from build123d import *

# Parameters (mm, degrees)
CORTE_EXTRUS_O1_DEPTH      = 51.902259282
CORTE_EXTRUS_O1_DEPTH_BACK = 51.902259282
ESBO_O2_R                  = 4.25


with BuildPart() as part:
    # Esboço1 → Revolução1 (revolve)
    with BuildSketch(Plane(origin=(0, 0, 0), x_dir=(0, 0, -1), z_dir=(1, 0, 0))):
        Polygon((15.5, 35.2), (15.5, 0), (24.5, 0), (26, 1.5), (26, 22.5), (22.5, 22.5), (22.5, 35.2), align=None)
    revolve(axis=Axis((0, 0, 0), (0, 1, 0)))

    # Esboço2 → Corte-extrusão1 (cut, two sides: drawn at the far end of the back side and taken through both)
    with BuildSketch(Plane.XY.offset(-CORTE_EXTRUS_O1_DEPTH_BACK)):
        with Locations((0, 9.5)):
            Circle(ESBO_O2_R)
    extrude(amount=CORTE_EXTRUS_O1_DEPTH + CORTE_EXTRUS_O1_DEPTH_BACK, mode=Mode.SUBTRACT)


solid = part.part
Model file for the job. Use its own axes, mm. A direction names the side the tool comes from. Give positions to 0.01 mm unless a question says otherwise; leave off trailing zeros. Write each loop counter-clockwise with the first axis right and the second up, starting at its lowest first coordinate (ties: lowest second). Pieces come first, ordered by that corner, then holes. Notation, with made-up numbers: M 81,-18 L 100,-18 A18 cw 100,16 Z; hole C 68,-14.75 d2. An arc over 180 degrees is marked long. One line per item, written item: value. Start each with the question number.
Q1. Two-plate mould, pull along X, no slides. Class faces 3 (the cylindrical face through (-4.656, 17.354, -14.784)), 4 (the flat face through (15, 35.2, 5)), 5 (the cylindrical face through (19.961, 28.939, -10.382)): +X half, -X half, draft (parallel to the pull), parting line (faces both ways), or undercut.
Q2. Saw through at B-B, the plane z = 0. Write the cut outline in (x, y), plus the area to 3 significant figures.
Q3. Probe probe 1 along Z at (x, y) = (0, 28); probe 2 along X at (y, z) = (18, -0.5); probe 3 along Y at (x, z) = (0, -20.5). List the from-to ranges inside material, lowest first. Write a range as [from, to].
Q4. Drop flat-ended pins along their axis: pin 1 Ø11 at (x, y) = (0, 9.5) entering from -Z; pin 2 Ø4 at (x, y) = (-4.5, 22.5) entering from -Z; pin 3 Ø10 at (y, z) = (8, -17.5) entering from +X; pin 4 Ø8 at (x, y) = (-17, 8) entering from +Z. Give the stop position or say it passes through.
Q5. 3-axis set-ups, long thin cutter, end or side, ignore diameter. For faces 1 (the flat face through (-19.4, 22.5, 11.7)), 2 (the cylindrical face through (-0.92, 5.35, -20.53)): which of +Z, -Z, +X, -X, +Y, -Y reach the whole face in a straight line?
Q6. Saw through at C-C, the plane y = 9.5. Write the cut outline in (x, z), plus the area to 3 significant figures.
Q7. Saw through at D-D, the plane y = 18. Write the cut outline in (x, z), plus the area to 3 significant figures.
Q8. Saw through at A-A, the plane x = 0. Write the cut outline in (y, z), plus the area to 3 significant figures.
Output values:
1. face 3: undercut
1. face 4: draft
1. face 5: parting line
2. outline: M -26,1.5 L -24.5,0 L -15.5,0 L -15.5,35.2 L -22.5,35.2 L -22.5,22.5 L -26,22.5 Z; M 15.5,0 L 24.5,0 L 26,1.5 L 26,22.5 L 22.5,22.5 L 22.5,35.2 L 15.5,35.2 Z
2. area: 648 mm²
3. probe 1: z = [-22.5, -15.5], [15.5, 22.5]
3. probe 2: x = [-26, -15.49], [15.49, 26]
3. probe 3: y = [0, 5.25], [13.75, 35.2]
4. pin 1: stops at z = -26
4. pin 2: stops at z = -25.88
4. pin 3: stops at x = 22.8
4. pin 4: stops at z = 22.52
5. face 1: +Y
5. face 2: +Z, -Z
6. outline: M -4.25,-25.65 L -4.25,-14.91 A15.5 cw -4.25,14.91 L -4.25,25.65 A26 ccw Z; M 4.25,-25.65 A26 ccw 4.25,25.65 L 4.25,14.91 A15.5 cw 4.25,-14.91 Z
6. area: 1,190 mm²
7. outline: C 0,0 d52; hole C 0,0 d31
7. area: 1,370 mm²
8. outline: M 0,-24.5 L 1.5,-26 L 5.25,-26 L 5.25,-15.5 L 0,-15.5 Z; M 0,15.5 L 5.25,15.5 L 5.25,26 L 1.5,26 L 0,24.5 Z; M 13.75,-26 L 22.5,-26 L 22.5,-22.5 L 35.2,-22.5 L 35.2,-15.5 L 13.75,-15.5 Z; M 13.75,15.5 L 35.2,15.5 L 35.2,22.5 L 22.5,22.5 L 22.5,26 L 13.75,26 Z
8. area: 470 mm²
